Part model, mm, in its own coordinate system. Face numbers are marked on the shaded views. Give positions to 0.01 mm unless a question says otherwise; leave off trailing zeros. Write each loop counter-clockwise with the first axis right and the second up, starting at its lowest first coordinate (ties: lowest second). Pieces come first, ordered by that corner, then holes. Notation, with made-up numbers: M -10,25.5 L 8,25.5 A22 ccw 8,58.5 Z; hole C 45.25,48 d6. An arc over 180 degrees is marked long. Write item = value, one per line. Start each with the question number.
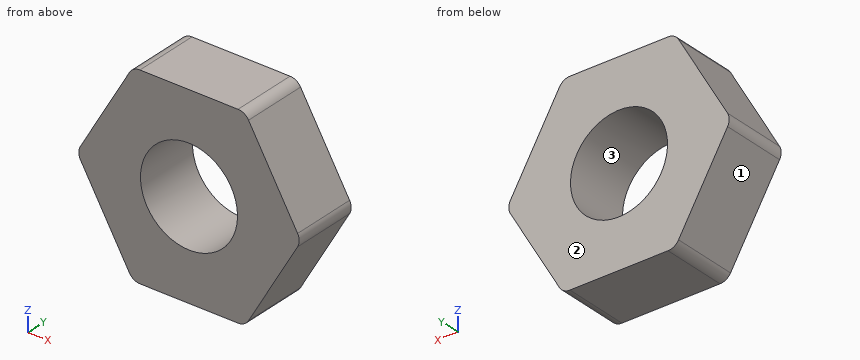
from build123d import *

# Parameters (mm, degrees)
SKETCH_1_R      = 2
EXTRUDE_1_DEPTH = 2.7
FILLET_1_R      = 0.5


with BuildPart() as part:
    # Эскиз1 → Бобышка-Вытянуть1 (new body)
    with BuildSketch(Plane(origin=(0, 0, 0), x_dir=(1, 0, 0), z_dir=(0, 1, 0))):
        Polygon((4.618802154, 0), (2.309401077, 4), (-2.309401077, 4), (-4.618802154, 0), (-2.309401077, -4), (2.309401077, -4), align=None)
        Circle(SKETCH_1_R, mode=Mode.SUBTRACT)
    extrude(amount=EXTRUDE_1_DEPTH)

    # Скругление1
    fillet_1_edges = [part.edges().sort_by_distance(p)[0] for p in [
        (2.309401077, 1.35, 4),
        (-2.309401077, 1.35, 4),
        (-4.618802154, 1.35, 0),
        (-2.309401077, 1.35, -4),
        (2.309401077, 1.35, -4),
        (4.618802154, 1.35, 0),
    ]]
    fillet(fillet_1_edges, radius=FILLET_1_R)


solid = part.part
Q1. Slice it at D-D (z = 3.25). Give the cut face in (x, y), and give its area (3 significant figures).
Q2. Slice it at A-A (x = 0). Give the cut face in (y, z).
Q3. Drop a flat-ended pin along its axis: P1, Ø1, axis at x = 3.5, y = 0.5, coming from the -Z side. Give the stop position or say it passes through.
Q4. Two-plate mould, pull along X, no slides. Class the marked faces 1, 2 and 3: +X half, -X half, draft (parallel to the pull), parting line (faces both ways), or undercut.
Q5. Probe line 1 along X through (y, z) = (0.9, 0); line 2 along Z through (x, y) = (0, 1.9); line 3 along Z through (x, y) = (-0.5, 1.6). List the from-to ranges inside material, lowest first.
Q6. Slice it at C-C (z = 0). Give the cut face in (x, y).
Q7. Slice it at B-B (y = 1.7). Give the cut face in (x, z).
Working result:
q1.outline = M -2.74,0 L 2.74,0 L 2.74,2.7 L -2.74,2.7 Z
q1.area = 14.8 mm2
q2.outline = M 0,-4 L 2.7,-4 L 2.7,-2 L 0,-2 Z; M 0,2 L 2.7,2 L 2.7,4 L 0,4 Z
q3.P1 = -2.8
q4.face_1 = -X half
q4.face_2 = draft
q4.face_3 = undercut
q5.line_1 = -4.54 to -2, 2 to 4.54
q5.line_2 = -4 to -2, 2 to 4
q5.line_3 = -4 to -1.94, 1.94 to 4
q6.outline = M -4.54,0 L -2,0 L -2,2.7 L -4.54,2.7 Z; M 2,0 L 4.54,0 L 4.54,2.7 L 2,2.7 Z
q7.outline = M -4.47,-0.25 L -2.45,-3.75 A0.5 ccw -2.02,-4 L 2.02,-4 A0.5 ccw 2.45,-3.75 L 4.47,-0.25 A0.5 ccw 4.47,0.25 L 2.45,3.75 A0.5 ccw 2.02,4 L -2.02,4 A0.5 ccw -2.45,3.75 L -4.47,0.25 A0.5 ccw Z; hole C 0,0 d4
